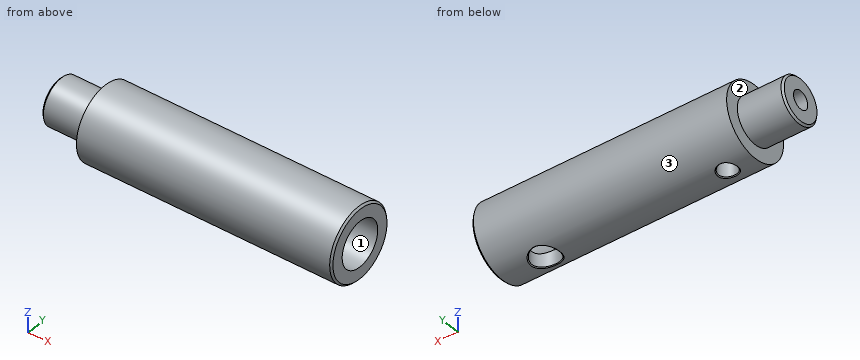
Autodesk Inventor part; units mm, degrees
ref_plane "YZ Plane" through (0, 0, 0) normal (1, 0, 0) x (0, 1, 0)
ref_plane "XZ Plane" through (0, 0, 0) normal (0, 1, 0) x (-1, 0, 0)
ref_plane "XY Plane" through (0, 0, 0) normal (0, 0, 1) x (1, 0, 0)
sketch "Skizze3" plane through (0, 0, 0) normal (0, 1, 0) x (-1, 0, 0)
  line L0 (-27.6589, 0) -> (27.6589, 0)
  line L1 (-14, 0) -> (-14, 4)
  line L2 (-14, 4) -> (14, 4)
  line L3 (14, 4) -> (14, 2.5)
  line L4 (14, 2.5) -> (19, 2.5)
  line L5 (19, 2.5) -> (19, 0)
  point P0 (0, 0)
  point P1 (0, 0)
  point P2 (14, 3.25)
  point P3 (0, 4)
  dimension "d4" = 8
  dimension "d5" = 5
  dimension "d6" = 5
  dimension "d7" = 28
revolve "Umdrehung1" add sketch "Skizze3" angle 360 about axis through (27.6589, 0, 0) along (-1, 0, 0)
sketch "Skizze4" plane through (14, 0, 0) normal (1, 0, 0) x (0, 0, -1)
  circle A0 centre (0, 0) radius 4
  point P0 (0, 0)
hole "Bohrung1" at (14, 0, 0) direction (-1, 0, 0) diameter 5 depth 22
hole "Bohrung2" at (14, 0, 0) direction (-1, 0, 0) diameter 2 depth 40
sketch "Skizze5" plane through (0, 0, 0) normal (0, 0, 1) x (1, 0, 0)
  line L0 (14, 4) -> (14, -4)
  line L1 (-19, 2.5) -> (-19, -2.5)
  line L2 (14, 0) -> (-19.3712, 0)
  line L3 (-14, 4) -> (-14, -4)
  point P0 (0, 0)
  point P1 (9, 0)
  point P2 (-11, 0)
  dimension "d23" = 3
  dimension "d24" = 5
hole "Bohrung3" at (-11, 0, 0) direction (0, 0, -1) diameter 2 depth 5
hole "Bohrung4" at (9, 0, 0) direction (0, 0, -1) diameter 3 depth 4
thread "Gewinde1"
thread "Gewinde2"
chamfer "Fase1" distance 0.1 angle 45 4 edges at (9.9974, -1.1203, -3.8399) (9.0005, 1.5, -3.7081) (8.0025, -1.1203, -3.8399) (-11.0007, 1, -3.873)
chamfer "Fase2" distance 0.2 angle 45 2 edges at (14, 0, -4) (-19, 0, -2.5)
properties part number "BT805_goteln20_22" material "Messing"
Work out the finished part from the listing and answer in its coordinate system (mm). Face numbers are marked on the shaded views. Give positions to 0.01 mm unless a question says otherwise; leave off trailing zeros. Loops run counter-clockwise (first coordinate to the right, second up) from the corner with the lowest first, then second, coordinate; pieces in that order, holes last. Notation, with made-up numbers: M -27.75,48.5 L -19.75,48.5 A36 cw -19.75,87.5 Z; hole C -36,64.25 d1. An arc over 180 degrees is marked long. Use CSV: the item, a comma, the result in double quotes.
1) Find section B-B on x = -16.5. Write down the section's boundary in (y, z), plus the area to 3 significant figures.
Answer:
outline,"C 0,0 d5; hole C 0,0 d2"
area,"16.5 mm^2"
2) Given P1, Ø2, axis at x = -13, y = -1.5, coming from the +Z side; P2, Ø1, axis at y = 0.5, z = -1.5, coming from the +X side; P3, Ø1.5, axis at x = 4, z = -0.5, coming from the -Y side; P4, Ø1.2, axis at x = -11, y = 0, coming from the -Z side, each flat-ended and moving along its own axis, determine where each tip first touches the part or whether it passes through.
Answer:
P1,"z = 3.97"
P2,"x = -8"
P3,"y = -4"
P4,"z = 0.8"
3) Consider L1, parallel to Z at x = -3, y = 0; L2, parallel to X at y = 0, z = -1.3; L3, parallel to Y at x = -13.25, z = 0. Determine where each line is inside the solid, lowest interval first.
Answer:
L1,"-4 to -2.5, 2.5 to 4"
L2,"-19 to -12, -10 to -8"
L3,"-4 to -1, 1 to 4"
4) Determine the mould class of the marked faces 1, 2 and 3 for opening direction Y: released by +Y, released by -Y, zero draft, split by the parting line, or undercut.
Answer:
face 1,"undercut"
face 2,"zero draft"
face 3,"split by the parting line"
5) Find section A-A on x = -5. Write down the section's boundary in (y, z).
Answer:
outline,"C 0,0 d8; hole C 0,0 d5"
